from build123d import *

# Parameters (mm, degrees)
SKETCH_1_W                  = 250
SKETCH_1_H                  = 250
EXTRUDE_1_DEPTH             = 65.5
SKETCH_2_W                  = 244
SKETCH_2_H                  = 62.5
CUT_EXTRUDE_1_DEPTH         = 286.161796179
SKETCH_3_W                  = 40
SKETCH_3_H                  = 40
CUT_EXTRUDE_2_DEPTH         = 287.410980935
CUT_EXTRUDE_3_DEPTH         = 287.410980935
SKETCH_5_W                  = 40
SKETCH_5_H                  = 40
CUT_EXTRUDE_4_DEPTH         = 287.410980935
CUT_EXTRUDE_5_DEPTH         = 288.080563605
HOLE_WIZARD_2_5_2_5_1_D     = 2.5
HOLE_WIZARD_2_5_2_5_2_D     = 2.5
HOLE_WIZARD_2_5_2_5_2_DEPTH = 3
HOLE_WIZARD_2_5_2_5_3_D     = 2.5
FILLET_1_R                  = 44.5
FILLET_2_R                  = 47.5


with BuildPart() as part:
    # Эскиз1 → Бобышка-Вытянуть1 (new body)
    with BuildSketch(Plane.XY.offset(56.5)):
        with Locations((0, 125)):
            Rectangle(SKETCH_1_W, SKETCH_1_H)
    extrude(amount=-EXTRUDE_1_DEPTH)

    # Эскиз2 → Вырез-Вытянуть1 (cut, through all)
    with BuildSketch(Plane.XZ):
        with Locations((0, 22.25)):
            Rectangle(SKETCH_2_W, SKETCH_2_H)
    extrude(amount=-CUT_EXTRUDE_1_DEPTH, mode=Mode.SUBTRACT)

    # Эскиз3 → Вырез-Вытянуть2 (cut, through all)
    with BuildSketch(Plane(origin=(0, 0, 53.5), x_dir=(-1, 0, 0), z_dir=(0, 0, -1))):
        with Locations((40, 202)):
            Rectangle(SKETCH_3_W, SKETCH_3_H)
    extrude(amount=-CUT_EXTRUDE_2_DEPTH, mode=Mode.SUBTRACT)

    # Эскиз4 → Вырез-Вытянуть3 (cut, through all)
    with BuildSketch(Plane(origin=(0, 0, 53.5), x_dir=(-1, 0, 0), z_dir=(0, 0, -1))):
        with BuildLine():
            Line((-50, 103), (-50, 43))
            ThreePointArc((-50, 43), (-40, 33), (-30, 43))
            Line((-30, 43), (-30, 103))
            ThreePointArc((-30, 103), (-40, 113), (-50, 103))
        make_face()
    extrude(amount=-CUT_EXTRUDE_3_DEPTH, mode=Mode.SUBTRACT)

    # Эскиз5 → Вырез-Вытянуть4 (cut, through all)
    with BuildSketch(Plane(origin=(0, 0, 53.5), x_dir=(-1, 0, 0), z_dir=(0, 0, -1))):
        with Locations((-40, 202)):
            Rectangle(SKETCH_5_W, SKETCH_5_H)
    extrude(amount=-CUT_EXTRUDE_4_DEPTH, mode=Mode.SUBTRACT)

    # Эскиз6 → Вырез-Вытянуть5 (cut, through all)
    with BuildSketch(Plane.XY.offset(56.5)):
        with BuildLine():
            Line((-30, 43), (-30, 103))
            ThreePointArc((-30, 103), (-40, 113), (-50, 103))
            Line((-50, 103), (-50, 43))
            ThreePointArc((-50, 43), (-40, 33), (-30, 43))
        make_face()
    extrude(amount=-CUT_EXTRUDE_5_DEPTH, mode=Mode.SUBTRACT)

    # Диаметр отверстия Ø2.5 (2.5)1 (through all)
    with Locations(Plane(origin=(0, 0, 53.5), x_dir=(-1, 0, 0), z_dir=(0, 0, -1))):
        with Locations((60, 166.5), (20, 235), (20, 166.5), (-20, 133.5), (-20, 15), (-40, 166.5), (-40, 15), (-60, 235), (-60, 166.5), (60, 55), (20, 93.5), (20, 55), (-20, 93.5), (-20, 55), (-60, 93.5), (-60, 55), (60, 93.5), (-60, 15), (-60, 133.5), (-40, 133.5), (-40, 235), (-20, 166.5), (-20, 235), (20, 15), (20, 133.5), (40, 15), (40, 133.5), (40, 166.5), (40, 235), (60, 15), (60, 133.5), (60, 235)):
            Hole(HOLE_WIZARD_2_5_2_5_1_D / 2)

    # Диаметр отверстия Ø2.5 (2.5)2
    with Locations(Plane.ZY.offset(-122)):
        with Locations((-3.5, 232), (-3.5, 18), (-3.5, 76), (-3.5, 133.5), (-3.5, 166.5)):
            Hole(HOLE_WIZARD_2_5_2_5_2_D / 2, depth=HOLE_WIZARD_2_5_2_5_2_DEPTH)

    # Диаметр отверстия Ø2.5 (2.5)3 (through all)
    with Locations(Plane(origin=(-122, 0, 0), x_dir=(0, 0, -1), z_dir=(1, 0, 0))):
        with Locations((3.5, 232), (3.5, 166.5), (3.5, 76), (3.5, 18), (3.5, 133.5)):
            Hole(HOLE_WIZARD_2_5_2_5_3_D / 2)

    # Скругление1
    fillet_1_edges = [part.edges().sort_by_distance(p)[0] for p in [
        (-122, 125, 53.5),
        (122, 125, 53.5),
    ]]
    fillet(fillet_1_edges, radius=FILLET_1_R)

    # Скругление2
    fillet_2_edges = [part.edges().sort_by_distance(p)[0] for p in [
        (125, 125, 56.5),
        (-125, 125, 56.5),
    ]]
    fillet(fillet_2_edges, radius=FILLET_2_R)


solid = part.part
Geometry: final body of the model. Coordinates: model frame, mm. A direction names the side the tool comes from. Round coordinates to 2 decimals unless told otherwise and drop trailing zeros. Loops run counter-clockwise (first coordinate to the right, second up) from the corner with the lowest first, then second, coordinate; pieces in that order, holes last. Notation, with made-up numbers: M 4.5,-13 L 53.5,-13 A27 ccw 53.5,13 Z; hole C 60,27.5 d1. An arc over 180 degrees is marked long. One line per question, with ' | ' between items.
(1) Pull-direction query (Y, two-part tool) for faces 4 (the flat face through (-10, 250, 55)), 5 (the cylindrical face through (-40, 113, 55)), 6 (the cylindrical face through (40, 113, 55)), 7 (the flat face through (-1, 123, 53.5)); classes: +Y half, -Y half, draft (parallel to the pull), parting line (faces both ways), or undercut.
Check result:
face 4: +Y half | face 5: undercut | face 6: undercut | face 7: draft
(2) Cut plane A-A on x = -27. Return the cut outline in (y, z).
Check result:
outline: M 0,53.5 L 182,53.5 L 182,56.5 L 0,56.5 Z; M 222,53.5 L 250,53.5 L 250,56.5 L 222,56.5 Z
(3) Material intervals for line 1 along Y through (x, z) = (-123.45, -3.5); line 2 along X through (y, z) = (183, 7); line 3 along X through (y, z) = (126, 33), sorted ascending. Write a range as from..to.
Check result:
line 1: y = 0..16.75, 19.25..74.75, 77.25..132.25, 134.75..165.25, 167.75..230.75, 233.25..250 | line 2: x = -125..-122, 122..125 | line 3: x = -118.49..-114.97, 114.97..118.49
(4) Cut plane D-D on y = 127.5. Return the cut outline in (x, z), plus the area to 3 significant figures.
Check result:
outline: M -125,-9 L -122,-9 L -122,9 A44.5 cw -77.5,53.5 L 77.5,53.5 A44.5 cw 122,9 L 122,-9 L 125,-9 L 125,9 A47.5 ccw 77.5,56.5 L -77.5,56.5 A47.5 ccw -125,9 Z | area: 1,010 mm2
(5) Cut plane C-C on y = 60. Return the cut outline in (x, z), plus the area to 3 significant figures.
Check result:
outline: M -125,-9 L -122,-9 L -122,9 A44.5 cw -77.5,53.5 L -50,53.5 L -50,56.5 L -77.5,56.5 A47.5 ccw -125,9 Z; M -30,53.5 L 30,53.5 L 30,56.5 L -30,56.5 Z; M 50,53.5 L 77.5,53.5 A44.5 cw 122,9 L 122,-9 L 125,-9 L 125,9 A47.5 ccw 77.5,56.5 L 50,56.5 Z | area: 887 mm2
(6) Contact query for flat-ended pins moving along their axis: P1, Ø1.5, axis at x = -40, y = 133.5, coming from the -Z side; P2, Ø3, axis at x = 88, y = 106, coming from the -Z side; P3, Ø10, axis at y = 45, z = 36, coming from the +X side; P4, Ø1.5, axis at y = 107.5, z = 27.5, coming from the -X side. Output: stop coordinate, or through.
Check result:
P1: passes through | P2: stops at z = 51.85 | P3: stops at x = 119.6 | P4: stops at x = -121.56
(7) Access query for faces 1 (the flat face through (-122, 123, 0)), 2 (the flat face through (-10, 0, 55)), 3 (the cylindrical face through (-40, 33, 55)). Directions: +Z, -Z, +X, -X, +Y, -Y. A direction counts if a zero-diameter tool reaches every point of the face in a straight line with its end or side. Return the directions, or none.
Check result:
face 1: -Z, +Y, -Y | face 2: +Z, -Z, +X, -X, -Y | face 3: +Z, -Z
(8) Cut plane B-B on z = 6. Return the cut outline in (x, y), plus the area to 3 significant figures.
Check result:
outline: M -125,0 L -122,0 L -122,250 L -125,250 Z; M 122,0 L 125,0 L 125,250 L 122,250 Z | area: 1,500 mm2
